Design review of the part built by this model. Coordinates are the model's own, in mm. A direction names the side the tool comes from. Give positions to 0.01 mm unless a question says otherwise; leave off trailing zeros. Order: outer loops, then holes, each group sorted by start corner. A loop starts at its lowest first (then second) coordinate and runs counter-clockwise, first axis right, second up.
```python
from build123d import *

# Parameters (mm, degrees)
SKETCH1_W           = 1.5
SKETCH1_H           = 21
SKETCH1_W_2         = 7.8
SKETCH1_H_2         = 8.247795839
BOSS_EXTRUDE1_DEPTH = 1.25


with BuildPart() as part:
    # Sketch1 → Boss-Extrude1 (new body)
    with BuildSketch(Plane(origin=(0, 0, 0), x_dir=(1, 0, 0), z_dir=(0, 1, 0))):
        with BuildLine():
            Line((0, 1), (0, 22.252194503))
            ThreePointArc((0, 22.252194503), (-0.051316702, 22.568422269), (-0.2, 22.852194503))
            Line((-0.2, 22.852194503), (-4.453950106, 28.524127978))
            ThreePointArc((-4.453950106, 28.524127978), (-4.539729418, 28.660021298), (-4.602633404, 28.807900212))
            Line((-4.602633404, 28.807900212), (-6, 33))
            Line((-6, 33), (-10.554092553, 33))
            Line((-10.554092553, 33), (-12.046049894, 28.524127978))
            ThreePointArc((-12.046049894, 28.524127978), (-12.10895388, 28.376249064), (-12.194733192, 28.240355744))
            Line((-12.194733192, 28.240355744), (-16.1, 23.033333333))
            ThreePointArc((-16.1, 23.033333333), (-16.248683298, 22.749561099), (-16.3, 22.433333333))
            Line((-16.3, 22.433333333), (-16.3, 1))
            ThreePointArc((-16.3, 1), (-16.007106781, 0.292893219), (-15.3, 0))
            Line((-15.3, 0), (-13.863109548, 0))
            ThreePointArc((-13.863109548, 0), (-13.600243992, -0.074674596), (-13.415895952, -0.276393202))
            Line((-13.415895952, -0.276393202), (-10.554092553, -6))
            Line((-10.554092553, -6), (-6, -6))
            Line((-6, -6), (-3.138196601, -0.276393202))
            ThreePointArc((-3.138196601, -0.276393202), (-2.953848562, -0.074674596), (-2.690983006, 0))
            Line((-2.690983006, 0), (-1, 0))
            ThreePointArc((-1, 0), (-0.292893219, 0.292893219), (0, 1))
        make_face()
        with Locations((-13.677046277, 11.25)):
            Rectangle(SKETCH1_W, SKETCH1_H, mode=Mode.SUBTRACT)
        with Locations((-2.877046277, 11.25)):
            Rectangle(SKETCH1_W, SKETCH1_H, mode=Mode.SUBTRACT)
        with Locations((-8.277046277, 16.12389792)):
            Rectangle(SKETCH1_W_2, SKETCH1_H_2, mode=Mode.SUBTRACT)
    extrude(amount=BOSS_EXTRUDE1_DEPTH)


solid = part.part
```
1. Machinability: for faces 4 (the face through (-5.3, 0.6, -30.9)), 5 (the face through (-2, 1, 0)), 6 (the face through (-15, 1, 0)), 7 (the face through (-11.29, 0.62, -30.79)), 8 (the face through (-14, 1, -0.75)), which of the approach directions +Z, -Z, +X, -X, +Y, -Y give a long, thin tool a straight path to every point of the face, cutting with its end or side? Answer none if there is none.
Recorded:
face 4: -Z, +X, +Y, -Y
face 5: +Z, +X, +Y, -Y
face 6: +Z, -X, +Y, -Y
face 7: -Z, -X, +Y, -Y
face 8: +Y, -Y
2. For pin 1 (3 mm diameter, centred on x = -9, z = -1.5, fed in from -Y), flat-tipped, find the tip position at first contact; note if it passes through.
Recorded:
pin 1: stops at y = 0
3. Take a section at D-D (z = -24). State the section outline as (x, y) points (3 decimals).
Recorded:
outline: (-15.375, 0) - (-1.061, 0) - (-1.061, 1.25) - (-15.375, 1.25) - close
4. Draft analysis for pull direction Z (two halves, no side actions). For faces 1 (the face through (-12.927, 1, -11)), 2 (the face through (-8, 1.25, -9)), 3 (the face through (-12.005, 0.616, 3.098)), state which applies: pulls with the +Z half, pulls with the -Z half, needs draft (parallel to the pull), parting line crosses it, or undercut.
Recorded:
face 1: undercut
face 2: needs draft
face 3: pulls with the +Z half
5. Take a section at B-B (y = 0.55). State how many separate pieces and enclosed holes the cut face has, then the cut area to 3 significant figures.
Recorded:
separate pieces: 1
enclosed holes: 3
area: 384 mm2
6. Take a section at C-C (z = -3.5). State the section outline as (x, y) points, then the cut area to 3 significant figures.
Recorded:
outline: (-16.3, 0) - (-14.43, 0) - (-14.43, 1.25) - (-16.3, 1.25) - close; (-12.93, 0) - (-3.63, 0) - (-3.63, 1.25) - (-12.93, 1.25) - close; (-2.13, 0) - (0, 0) - (0, 1.25) - (-2.13, 1.25) - close
area: 16.6 mm2
7. For line 1 along X through (y, z) = (0.55, -11); line 2 along X through (y, z) = (0.65, -14.5); line 3 along Z through (x, y) = (-10.25, 1), list the stretches that pass through material, from the lowest coordinate up.
Recorded:
line 1: x = -16.3 to -14.43, -12.93 to -3.63, -2.13 to 0
line 2: x = -16.3 to -14.43, -12.93 to -12.18, -4.38 to -3.63, -2.13 to 0
line 3: z = -33 to -20.25, -12 to 6
8. Take a section at A-A (x = -9.5). State the section outline as (y, z) points, then the cut area to 3 significant figures.
Recorded:
outline: (0, -33) - (1.25, -33) - (1.25, -20.25) - (0, -20.25) - close; (0, -12) - (1.25, -12) - (1.25, 6) - (0, 6) - close
area: 38.4 mm2
